Could you check a few things on this model? Use its own coordinates, in mm. Face numbers are marked on the shaded views. A direction names the side the tool comes from. Round coordinates to 2 decimals unless told otherwise and drop trailing zeros. Write each loop counter-clockwise with the first axis right and the second up, starting at its lowest first coordinate (ties: lowest second). Pieces come first, ordered by that corner, then holes. Notation, with made-up numbers: (-7, -11.5) - (41, -11.5) arc R20 ccw to (41, 18.5) - close; hole circle Ø8 at (7.5, 59). An arc over 180 degrees is marked (long way). Put each result on its own line as item: value.
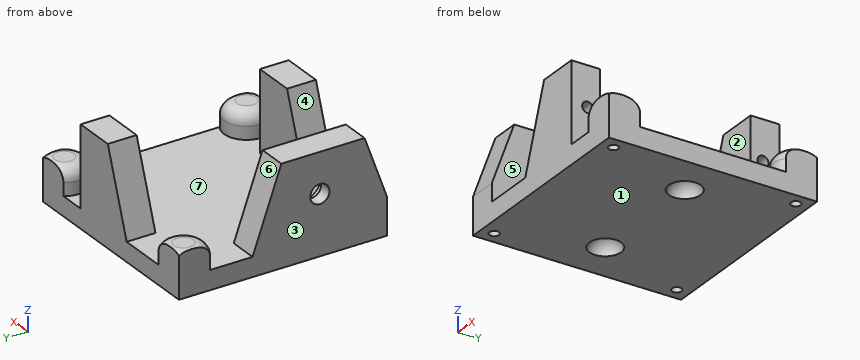
from build123d import *

# Parameters (mm, degrees)
EXTRUDE_635_DEPTH      = 6.25
SKETCH_691_R           = 0.85
CUT_EXTRUDE_915_DEPTH  = 5.5
SKETCH_5_W             = 2.5
SKETCH_5_H             = 8
CUT_EXTRUDE_1224_DEPTH = 4.5
SKETCH_1_W             = 32.5
SKETCH_1_H             = 32.5
EXTRUDE_1784_DEPTH     = 3
SKETCH_4_R             = 1.5
CUT_EXTRUDE_2137_DEPTH = 34.669348078
SKETCH_9_R             = 2.5
CUT_EXTRUDE_4617_DEPTH = 2.5
FILLET_3_R             = 2.5
SKETCH_10_W            = 12.5
SKETCH_10_H            = 12.5
CUT_EXTRUDE_5023_DEPTH = 39.52353177
CUT_EXTRUDE_5450_REACH = 39.495
SKETCH_13_W            = 12.5
SKETCH_13_H            = 16
SKETCH_13_H_2          = 3.5
CHAMFER_3_SIZE         = 4.5
CHAMFER_3_SIZE_2       = 12.5
CHAMFER_4_SIZE2        = 12.5
CHAMFER_4_SIZE         = 4.5
SKETCH_15_R            = 0.75
CUT_EXTRUDE_5895_DEPTH = 7
EXTRUDE_6483_DEPTH     = 4
SKETCH_17_R            = 3.25
CUT_EXTRUDE_7051_DEPTH = 2.5


with BuildPart() as part:
    # Эскиз2 → Extrude 635 (new, symmetric)
    with BuildSketch(Plane.XY):
        Polygon((9.5, 16.25), (-14, 16.25), (-14, -16.25), (9.5, -16.25), (9.5, -11.75), (-9.5, -11.75), (-9.5, 11.75), (9.5, 11.75), align=None)
    extrude(amount=EXTRUDE_635_DEPTH, both=True)

    # Sketch 691 → Cut-Extrude 915 (cut)
    with BuildSketch(Plane(origin=(9.5, 0, 0), x_dir=(0, 0, -1), z_dir=(1, 0, 0))):
        with Locations((0, 13.7)):
            Circle(SKETCH_691_R)
        with Locations((0, -13.7)):
            Circle(SKETCH_691_R)
    extrude(amount=-CUT_EXTRUDE_915_DEPTH, mode=Mode.SUBTRACT)

    # Эскиз5 → Cut-Extrude 1224 (cut)
    with BuildSketch(Plane.XZ.offset(11.75)):
        with Locations((-4.2, 2.25)):
            Rectangle(SKETCH_5_W, SKETCH_5_H)
    extrude(amount=CUT_EXTRUDE_1224_DEPTH, mode=Mode.SUBTRACT)

    # Эскиз1 → Extrude 1784 (add)
    with BuildSketch(Plane(origin=(0, 0, -6.25), x_dir=(-1, 0, 0), z_dir=(0, 0, -1))):
        with Locations((-2.25, 0)):
            Rectangle(SKETCH_1_W, SKETCH_1_H)
    extrude(amount=EXTRUDE_1784_DEPTH)

    # Эскиз4 → Cut-Extrude 2137 (cut, through all)
    with BuildSketch(Plane(origin=(-9.5, 0, 0), x_dir=(0, 0, -1), z_dir=(1, 0, 0))):
        with Locations(Location((0, -5.77, 0), (0, 0, 90))):
            Circle(SKETCH_4_R)
    extrude(amount=-CUT_EXTRUDE_2137_DEPTH, mode=Mode.SUBTRACT)

    # Эскиз9 → Cut-Extrude 4617 (cut)
    with BuildSketch(Plane(origin=(0, 0, -9.25), x_dir=(-1, 0, 0), z_dir=(0, 0, -1))):
        with Locations((-11.75, 0)):
            Circle(SKETCH_9_R)
        with Locations((7.25, 0)):
            Circle(SKETCH_9_R)
    extrude(amount=-CUT_EXTRUDE_4617_DEPTH, mode=Mode.SUBTRACT)

    # Скругление3
    fillet_3_edges = [part.edges().sort_by_distance(p)[0] for p in [
        (14.25, 0, -6.75),
        (-4.75, 0, -6.75),
    ]]
    fillet(fillet_3_edges, radius=FILLET_3_R - 0.0001)  # a hair under: the kernel refuses the full size

    # Эскиз10 → Cut-Extrude 5023 (cut, through all)
    with BuildSketch(Plane(origin=(0, 16.25, 0), x_dir=(1, 0, 0), z_dir=(0, 1, 0))):
        with Locations((-3.25, 0)):
            Rectangle(SKETCH_10_W, SKETCH_10_H)
    extrude(amount=-CUT_EXTRUDE_5023_DEPTH, mode=Mode.SUBTRACT)

    # Эскиз13 → Cut-Extrude 5450 (cut, up to next)
    with BuildSketch(Plane.ZY.offset(14), mode=Mode.PRIVATE) as cut_extrude_5450_sk1:
        with Locations((0, 8.25)):
            Rectangle(SKETCH_13_W, SKETCH_13_H)
    cut_extrude_5450_tool1 = extrude(cut_extrude_5450_sk1.sketch, amount=-CUT_EXTRUDE_5450_REACH, mode=Mode.PRIVATE) & part.part
    # Эскиз13 → Cut-Extrude 5450 (cut, up to next)
    with BuildSketch(Plane.ZY.offset(14), mode=Mode.PRIVATE) as cut_extrude_5450_sk2:
        with Locations((0, -14.5)):
            Rectangle(SKETCH_13_W, SKETCH_13_H_2)
    cut_extrude_5450_tool2 = extrude(cut_extrude_5450_sk2.sketch, amount=-CUT_EXTRUDE_5450_REACH, mode=Mode.PRIVATE) & part.part
    add(cut_extrude_5450_tool1.solids().sort_by_distance((-14, 8.25, 0))[0], mode=Mode.SUBTRACT)
    add(cut_extrude_5450_tool2.solids().sort_by_distance((-14, -14.5, 0))[0], mode=Mode.SUBTRACT)

    # Фаска3
    # the kernel refuses this chamfer: 12.5, 4.5 mm, written as the material it adds along each edge
    with BuildSketch(Plane(origin=(3, 16.25, -6.25), x_dir=(-1, 0, 0), z_dir=(0, -1, 0))) as chamfer_3_piece_1:
        Polygon((CHAMFER_3_SIZE, 0), (0, -CHAMFER_3_SIZE_2), (0, 0), align=None)
    extrude(amount=4.5)
    with BuildSketch(Plane(origin=(3, 48.678873385, -6.25), x_dir=(-1, 0, 0), z_dir=(0, -1, 0))) as chamfer_3_piece_2_section:
        Polygon((CHAMFER_3_SIZE, 0), (0, -CHAMFER_3_SIZE_2), (0, 0), align=None)
    chamfer_3_piece_2 = extrude(amount=69.357746771, mode=Mode.PRIVATE)
    chamfer_3_piece_2 = split(chamfer_3_piece_2, bisect_by=Plane(origin=(3, -16.25, -6.25), z_dir=(0, 1, 0)), keep=Keep.TOP, mode=Mode.PRIVATE)
    chamfer_3_piece_2 = split(chamfer_3_piece_2, bisect_by=Plane(origin=(3, -11.75, -6.25), z_dir=(0, -1, 0)), keep=Keep.TOP, mode=Mode.PRIVATE)
    add(chamfer_3_piece_2)
    with BuildSketch(Plane(origin=(3, 20.678873385, -6.25), x_dir=(0, 0, 1), z_dir=(0, -1, 0))) as chamfer_3_piece_3_section:
        Polygon((CHAMFER_3_SIZE_2, 0), (0, CHAMFER_3_SIZE), (0, 0), align=None)
    chamfer_3_piece_3 = extrude(amount=69.357746771, mode=Mode.PRIVATE)
    chamfer_3_piece_3 = split(chamfer_3_piece_3, bisect_by=Plane(origin=(3, 11.75, -6.25), z_dir=(0, 1, 0)), keep=Keep.TOP, mode=Mode.PRIVATE)
    chamfer_3_piece_3 = split(chamfer_3_piece_3, bisect_by=Plane(origin=(3, 16.25, -6.25), z_dir=(0, -1, 0)), keep=Keep.TOP, mode=Mode.PRIVATE)
    add(chamfer_3_piece_3)
    with BuildSketch(Plane(origin=(3, -11.75, -6.25), x_dir=(0, 0, 1), z_dir=(0, -1, 0))) as chamfer_3_piece_4:
        Polygon((CHAMFER_3_SIZE_2, 0), (0, CHAMFER_3_SIZE), (0, 0), align=None)
    extrude(amount=4.5)
    with BuildSketch(Plane(origin=(-14, -12.75, -6.25), x_dir=(0, -1, 0), z_dir=(1, 0, 0))) as chamfer_3_piece_5_section:
        Polygon((CHAMFER_3_SIZE, 0), (0, -CHAMFER_3_SIZE_2), (0, 0), align=None)
    chamfer_3_piece_5 = extrude(amount=4.5, mode=Mode.PRIVATE)
    chamfer_3_piece_5 = split(chamfer_3_piece_5, bisect_by=Plane(origin=(-14, -16.25, -6.25), z_dir=(0, 1, 0)), keep=Keep.TOP, mode=Mode.PRIVATE)
    add(chamfer_3_piece_5)

    # Фаска4
    chamfer_4_edges = [part.edges().sort_by_distance(p)[0] for p in [
        (-11.75, 0.25, -6.25),
    ]]
    chamfer_4_side = [part.faces().sort_by_distance(p)[0] for p in [
        (-11.75, 0.34, -6.25),
    ]]
    chamfer(chamfer_4_edges, length=CHAMFER_4_SIZE - 0.0001, length2=CHAMFER_4_SIZE2 - 0.0001, reference=chamfer_4_side[0])  # a hair under: the kernel refuses the full size

    # Эскиз15 → Cut-Extrude 5895 (cut)
    with BuildSketch(Plane(origin=(0, 0, -9.25), x_dir=(-1, 0, 0), z_dir=(0, 0, -1))):
        with Locations((12, -14.25)):
            Circle(SKETCH_15_R)
        with Locations((12, 14.25)):
            Circle(SKETCH_15_R)
        with Locations((-16.5, 14.25)):
            Circle(SKETCH_15_R)
        with Locations((-16.5, -14.25)):
            Circle(SKETCH_15_R)
    extrude(amount=-CUT_EXTRUDE_5895_DEPTH, mode=Mode.SUBTRACT)

    # Эскиз16 → Extrude 6483 (add)
    with BuildSketch(Plane.XY.offset(-6.25)):
        with BuildLine():
            Line((-14, 11.377718677), (-14, 16.25))
            Line((-14, 16.25), (-9.127718677, 16.25))
            ThreePointArc((-9.127718677, 16.25), (-9.525126266, 11.775126266), (-14, 11.377718677))
        make_face()
        with BuildLine():
            Line((13.627718677, 16.25), (18.5, 16.25))
            Line((18.5, 16.25), (18.5, 11.377718677))
            ThreePointArc((18.5, 11.377718677), (14.025126266, 11.775126266), (13.627718677, 16.25))
        make_face()
        with BuildLine():
            Line((18.5, -11.377718677), (18.5, -16.25))
            Line((18.5, -16.25), (13.627718677, -16.25))
            ThreePointArc((13.627718677, -16.25), (14.025126266, -11.775126266), (18.5, -11.377718677))
        make_face()
    extrude(amount=EXTRUDE_6483_DEPTH)

    # Скругление4: read off the stored shape, not the designer's step
    # Скругление4 outline → Скругление4 (revolve, cut)
    with BuildSketch(Plane(origin=(16.5, 14.25, 0), x_dir=(1, 0, 0), z_dir=(0, -1, 0))):
        with BuildLine():
            ThreePointArc((1.5, -2.25), (2.914213562, -2.835786438), (3.5, -4.25))
            Line((3.5, -4.25), (3.5, -2.25))
            Line((3.5, -2.25), (1.5, -2.25))
        make_face()
    revolve(axis=Axis((16.5, 14.25, 0), (0, 0, 1)), mode=Mode.SUBTRACT)

    # Fillet 4 2 outline → Fillet 4 2 (revolve, cut)
    with BuildSketch(Plane(origin=(-12, 14.25, 0), x_dir=(1, 0, 0), z_dir=(0, -1, 0))):
        with BuildLine():
            ThreePointArc((1.5, -2.25), (2.914213562, -2.835786438), (3.5, -4.25))
            Line((3.5, -4.25), (3.5, -2.25))
            Line((3.5, -2.25), (1.5, -2.25))
        make_face()
    revolve(axis=Axis((-12, 14.25, 0), (0, 0, 1)), mode=Mode.SUBTRACT)

    # Fillet 4 3 outline → Fillet 4 3 (revolve, cut)
    with BuildSketch(Plane(origin=(16.5, -14.25, 0), x_dir=(1, 0, 0), z_dir=(0, -1, 0))):
        with BuildLine():
            ThreePointArc((1.5, -2.25), (2.914213562, -2.835786438), (3.5, -4.25))
            Line((3.5, -4.25), (3.5, -2.25))
            Line((3.5, -2.25), (1.5, -2.25))
        make_face()
    revolve(axis=Axis((16.5, -14.25, 0), (0, 0, 1)), mode=Mode.SUBTRACT)

    # Эскиз17 → Cut-Extrude 7051 (cut)
    with BuildSketch(Plane(origin=(-9.5, 0, 0), x_dir=(0, 0, -1), z_dir=(1, 0, 0))):
        with Locations((0, -5.77)):
            Circle(SKETCH_17_R)
    extrude(amount=-CUT_EXTRUDE_7051_DEPTH, mode=Mode.SUBTRACT)


solid = part.part
(1) Imagine slicing it at C-C, the plane x = 1.5. List the corners of the cut face in (y, z) for me.
Values found:
outline: (-16.25, -9.25) - (16.25, -9.25) - (16.25, 2.08) - (11.75, 2.08) - (11.75, -6.25) - (-11.75, -6.25) - (-11.75, 2.08) - (-16.25, 2.08) - close
(2) Please list where these lines run through material, in increasing order: probe 1 along Y at (x, z) = (16.5, -7.7); probe 2 along Y at (x, z) = (7.5, -2.5); probe 3 along Y at (x, z) = (9, 0.75). Write a range as from..to.
Values found:
probe 1: y = -16.25..-15, -13.5..13.5, 15..16.25
probe 2: y = -16.25..-11.75, 11.75..16.25
probe 3: y = -16.25..-14.1, -13.3..-11.75, 11.75..13.3, 14.1..16.25
(3) I'm going to push flat-ended pins straight in: pin 1 (6 mm diameter, centred on x = 13.5, z = -0.5, fed in from +Y); pin 2 (1.5 mm diameter, centred on x = 16, y = 14.5, fed in from +Z); pin 3 (6 mm diameter, centred on x = -5.5, z = -2, fed in from +Y); pin 4 (8 mm diameter, centred on x = -6, z = 3.5, fed in from -Y). Where does each tip first touch, or does it pass through?
Values found:
pin 1: stops at y = 16.25
pin 2: stops at z = -2.25
pin 3: passes through
pin 4: stops at y = -14.44
(4) Imagine slicing it at B-B, the plane z = 5.25. List the corners of the cut face in (x, y) for me.
Values found:
outline: (-14, -13.11) - (-9.5, -13.11) - (-9.5, 0.61) - (-14, 0.61) - close; (2.64, -16.25) - (9.5, -16.25) - (9.5, -11.75) - (2.64, -11.75) - close; (2.64, 11.75) - (9.5, 11.75) - (9.5, 16.25) - (2.64, 16.25) - close
(5) Imagine slicing it at A-A, the plane z = -5.75. List the corners of the cut face in (x, y) for me, then the cut area to 3 significant figures.
Values found:
outline: (-14, -16.25) - (-9.5, -16.25) - (-9.5, 4.57) - (-14, 4.57) - close; (-14, 11.38) arc R3.5 ccw to (-9.13, 16.25) - (-14, 16.25) - close; (-1.32, -16.25) - (9.5, -16.25) - (9.5, -11.75) - (-1.32, -11.75) - close; (-1.32, 11.75) - (9.5, 11.75) - (9.5, 16.25) - (-1.32, 16.25) - close; (13.63, -16.25) - (18.5, -16.25) - (18.5, -11.38) arc R3.5 ccw to start; (13.63, 16.25) arc R3.5 ccw to (18.5, 11.38) - (18.5, 16.25) - close; hole circle Ø1.5 at (-12, -14.25)
area: 270 mm^2
(6) If we mould it in two halves opening along X, with no side actions, what happens to the marked faces 1, 2 and 3? For each: pulls with the +X half, pulls with the -X half, needs draft (parallel to the pull), parting line crosses it, or undercut.
Values found:
face 1: needs draft
face 2: undercut
face 3: pulls with the -X half
(7) For the marked faces 4, 5, 6 and 7, which set-ups out of +Z, -Z, +X, -X, +Y, -Y let a thin tool reach every point of the face, with its end or its side?
Values found:
face 4: +Z, +Y, -Y
face 5: +Z, -Y
face 6: +Z, +X, -X
face 7: +Z
(8) Imagine slicing it at D-D, the plane y = -3. List the corners of the cut face in (x, z) for me.
Values found:
outline: (-14, -9.25) - (18.5, -9.25) - (18.5, -6.25) - (-9.5, -6.25) - (-9.5, -1.7) - (-12, -1.7) - (-12, 1.7) - (-9.5, 1.7) - (-9.5, 6.25) - (-14, 6.25) - close
